CAD build for the part. Positions are in the model's coordinates, mm. A direction names the side the tool comes from. Give positions to 0.01 mm unless a question says otherwise; leave off trailing zeros. Loops run counter-clockwise (first coordinate to the right, second up) from the corner with the lowest first, then second, coordinate; pieces in that order, holes last.
Item 1: Saw through at A-A on z = -45. Give the cut face in (x, y), plus the area to 3 significant figures.
Item 2: Probe probe 1 along Z at (x, y) = (-17.5, 6); probe 2 along X at (y, z) = (2.5, -69); probe 3 along Z at (x, y) = (-29, 1.25). List the from-to ranges inside material, lowest first.
Item 3: Which spindle directions (+Z, -Z, +X, -X, +Y, -Y) get a long thin tool onto all of the face, cutting with end or side? Do faces 1 (the flat face through (12.5, 4, -8)), 2 (the flat face through (-35, 4, -10)), 3 (the flat face through (60.416, 3.944, -12.371)). Say none if no direction does.
Item 4: Mould opens along Z. For faces 4 (the flat face through (-57.5, 4, -45)), 5 (the flat face through (0, 4, -15)), 6 (the flat face through (-1, 0, -21)) say: released by +Z, released by -Z, zero draft, split by the parting line, or undercut.
Item 5: Saw through at D-D on y = 4.75. Give the number of separate pieces and of enclosed holes in the cut face, plus the area to 3 significant figures.
Item 6: Drop flat-ended pins along their axis: P1, Ø4, axis at x = 13.5, y = 6, coming from the +Z side; P2, Ø2.5, axis at x = -17.5, z = -5, coming from the -Y side; P3, Ø4, axis at y = 4, z = -6, coming from the +X side; P4, Ø2.5, axis at y = 5.5, z = -7, coming from the -X side. Give the stop position or say it passes through.
Item 7: Saw through at B-B on x = -37.5. Give the cut face in (y, z), plus the area to 3 significant figures.
Item 8: Saw through at C-C on x = 17.5. Give the cut face in (y, z).
from build123d import *

# Parameters (mm, degrees)
SKETCH_1_R      = 1.6
EXTRUDE_1_DEPTH = 8
FILLET_1_R      = 1.6


with BuildPart() as part:
    # 草图1 → 凸台-拉伸1 (new body)
    with BuildSketch(Plane(origin=(0, 0, 0), x_dir=(1, 0, 0), z_dir=(0, 1, 0))):
        Polygon((-67.5, 74), (-67.5, 24.641016151), (-53.273502692, 0), (-12.5, 0), (-12.5, 15), (12.5, 15), (12.5, 0), (53.273502692, 0), (67.5, 24.641016151), (67.5, 74), align=None)
        with Locations(Location((17.5, 5, 0), (0, 0, 270))):
            Circle(SKETCH_1_R, mode=Mode.SUBTRACT)
        with Locations(Location((-62.5, 45, 0), (0, 0, 270))):
            Circle(SKETCH_1_R, mode=Mode.SUBTRACT)
        with Locations(Location((17.5, 69, 0), (0, 0, 270))):
            Circle(SKETCH_1_R, mode=Mode.SUBTRACT)
        with Locations(Location((-17.5, 5, 0), (0, 0, 90))):
            Circle(SKETCH_1_R, mode=Mode.SUBTRACT)
        with Locations(Location((-17.5, 69, 0), (0, 0, 90))):
            Circle(SKETCH_1_R, mode=Mode.SUBTRACT)
        with Locations(Location((62.5, 45, 0), (0, 0, 90))):
            Circle(SKETCH_1_R, mode=Mode.SUBTRACT)
        Polygon((-57.5, 27.320508076), (-57.5, 64), (57.5, 64), (57.5, 27.320508076), (47.5, 10), (22.5, 10), (22.5, 25), (-22.5, 25), (-22.5, 10), (-47.5, 10), align=None, mode=Mode.SUBTRACT)
    extrude(amount=EXTRUDE_1_DEPTH)

    # 圆角1
    fillet_1_edges = [part.edges().sort_by_distance(p)[0] for p in [
        (67.5, 4, -74),
        (67.5, 4, -24.641016151),
        (53.273502692, 4, 0),
        (12.5, 4, 0),
        (12.5, 4, -15),
        (-12.5, 4, -15),
        (-12.5, 4, 0),
        (-53.273502692, 4, 0),
        (-67.5, 4, -24.641016151),
        (-67.5, 4, -74),
        (57.5, 4, -27.320508076),
        (57.5, 4, -64),
        (-57.5, 4, -64),
        (-57.5, 4, -27.320508076),
        (-47.5, 4, -10),
        (-22.5, 4, -10),
        (-22.5, 4, -25),
        (22.5, 4, -25),
        (22.5, 4, -10),
        (47.5, 4, -10),
    ]]
    fillet(fillet_1_edges, radius=FILLET_1_R)


solid = part.part
Results below:
1. outline: (-67.5, 0) - (-64.1, 0) - (-64.1, 8) - (-67.5, 8) - close; (-60.9, 0) - (-57.5, 0) - (-57.5, 8) - (-60.9, 8) - close; (57.5, 0) - (60.9, 0) - (60.9, 8) - (57.5, 8) - close; (64.1, 0) - (67.5, 0) - (67.5, 8) - (64.1, 8) - close
1. area: 109 mm2
2. probe 1: z = -74 to -70.6, -67.4 to -64, -25 to -6.6, -3.4 to 0
2. probe 2: x = -67.5 to -19.1, -15.9 to 15.9, 19.1 to 67.5
2. probe 3: z = -74 to -64, -10 to 0
3. face 1: +Z, +Y, -Y
3. face 2: +Y, -Y
3. face 3: +Z, +X, +Y, -Y
4. face 4: undercut
4. face 5: released by +Z
4. face 6: zero draft
5. separate pieces: 1
5. enclosed holes: 7
5. area: 3,850 mm2
6. P1: stops at z = 0
6. P2: passes through
6. P3: stops at x = 57.89
6. P4: stops at x = -58.04
7. outline: (0, -74) - (8, -74) - (8, -64) - (0, -64) - close; (0, -10) - (8, -10) - (8, 0) - (0, 0) - close
7. area: 160 mm2
8. outline: (0, -74) - (8, -74) - (8, -70.6) - (0, -70.6) - close; (0, -67.4) - (8, -67.4) - (8, -64) - (0, -64) - close; (0, -25) - (8, -25) - (8, -6.6) - (0, -6.6) - close; (0, -3.4) - (8, -3.4) - (8, 0) - (0, 0) - close
